from build123d import *

# Parameters (mm, degrees)
SKETCH2_W           = 124
SKETCH2_H           = 62
SKETCH2_R           = 1.55
SKETCH2_W_2         = 26.6
SKETCH2_H_2         = 14.6
SKETCH2_R_2         = 3.75
SKETCH2_R_3         = 8.3
SKETCH2_R_4         = 8.2
BOSS_EXTRUDE1_DEPTH = 4
CHAMFER1_SIZE       = 1.5
CHAMFER2_SIZE       = 1
SKETCH2_3_R         = 0.8
BOSS_EXTRUDE2_DEPTH = 3.5
FILLET1_R           = 0.8
CUT_EXTRUDE1_START  = 3
SKETCH2_4_W         = 28
SKETCH2_4_H         = 28.35
SKETCH2_4_R         = 0.8
SKETCH2_4_W_2       = 26.6
SKETCH2_4_H_2       = 14.6
CUT_EXTRUDE1_DEPTH  = 3
CHAMFER3_SIZE       = 1
SKETCH2_5_W         = 13.2
SKETCH2_5_H         = 14
CUT_EXTRUDE4_DEPTH  = 1.5


with BuildPart() as part:
    # Sketch2 → Boss-Extrude1 (new body)
    with BuildSketch(Plane(origin=(0, 0, 0), x_dir=(1, 0, 0), z_dir=(0, 1, 0))):
        with Locations((62, 31)):
            Rectangle(SKETCH2_W, SKETCH2_H)
        with Locations(Location((4.5, 4.5, 0), (0, 0, 270))):
            Circle(SKETCH2_R, mode=Mode.SUBTRACT)
        with Locations(Location((119.5, 4.5, 0), (0, 0, 270))):
            Circle(SKETCH2_R, mode=Mode.SUBTRACT)
        with Locations((28.239743387, 41.89740921)):
            Rectangle(SKETCH2_W_2, SKETCH2_H_2, mode=Mode.SUBTRACT)
        with Locations(Location((4.5, 57.5, 0), (0, 0, 270))):
            Circle(SKETCH2_R, mode=Mode.SUBTRACT)
        with Locations(Location((67.078277823, 40.203161161, 0), (0, 0, 270))):
            Circle(SKETCH2_R_2, mode=Mode.SUBTRACT)
        with Locations(Location((119.5, 57.5, 0), (0, 0, 270))):
            Circle(SKETCH2_R, mode=Mode.SUBTRACT)
        with Locations(Location((102.593331931, 31, 0), (0, 0, 270))):
            Circle(SKETCH2_R_3, mode=Mode.SUBTRACT)
        with BuildLine():
            ThreePointArc((79.454234541, 11.660627935), (68.529234541, 14.839562505), (79.454234541, 18.018497075))
            Line((79.454234541, 18.018497075), (79.454234541, 11.660627935))
        make_face(mode=Mode.SUBTRACT)
        with Locations(Location((48.846547615, 14.839562505, 0), (0, 0, 270))):
            Circle(SKETCH2_R_4, mode=Mode.SUBTRACT)
        with Locations(Location((23.171087178, 14.839562505, 0), (0, 0, 270))):
            Circle(SKETCH2_R_4, mode=Mode.SUBTRACT)
    extrude(amount=BOSS_EXTRUDE1_DEPTH)

    # Chamfer1
    chamfer1_edges = [part.edges().sort_by_distance(p)[0] for p in [
        (62, 4, 0),
        (124, 4, -31),
        (62, 4, -62),
        (0, 4, -31),
    ]]
    chamfer(chamfer1_edges, length=CHAMFER1_SIZE)

    # Chamfer2
    chamfer2_edges = [part.edges().sort_by_distance(p)[0] for p in [
        (119.5, 0, -59.05),
        (4.5, 4, -6.05),
        (119.5, 4, -59.05),
        (119.5, 4, -6.05),
        (4.5, 4, -59.05),
    ]]
    chamfer(chamfer2_edges, length=CHAMFER2_SIZE)

    # Sketch2<3> → Boss-Extrude2 (add)
    with BuildSketch(Plane(origin=(0, 0, 0), x_dir=(1, 0, 0), z_dir=(0, 1, 0))):
        with Locations(Location((16.679743387, 28.409287577, 0), (0, 0, 270))):
            Circle(SKETCH2_3_R)
        with Locations(Location((16.679743387, 51.709287577, 0), (0, 0, 270))):
            Circle(SKETCH2_3_R)
        with Locations(Location((39.799743387, 28.409287577, 0), (0, 0, 270))):
            Circle(SKETCH2_3_R)
        with Locations(Location((39.799743387, 51.709287577, 0), (0, 0, 270))):
            Circle(SKETCH2_3_R)
    extrude(amount=-BOSS_EXTRUDE2_DEPTH)

    # Fillet1
    fillet1_edges = [part.edges().sort_by_distance(p)[0] for p in [
        (39.799743387, -3.5, -29.209287577),
        (39.799743387, -3.5, -52.509287577),
        (16.679743387, -3.5, -29.209287577),
        (16.679743387, -3.5, -52.509287577),
    ]]
    fillet(fillet1_edges, radius=FILLET1_R)

    # Sketch2<4> → Cut-Extrude1 (cut)
    with BuildSketch(Plane(origin=(0, 0, 0), x_dir=(1, 0, 0), z_dir=(0, 1, 0)).offset(CUT_EXTRUDE1_START)):
        with Locations((28.239743387, 39.62240921)):
            Rectangle(SKETCH2_4_W, SKETCH2_4_H)
        with Locations(Location((16.679743387, 51.709287577, 0), (0, 0, 270))):
            Circle(SKETCH2_4_R, mode=Mode.SUBTRACT)
        with Locations(Location((16.679743387, 28.409287577, 0), (0, 0, 270))):
            Circle(SKETCH2_4_R, mode=Mode.SUBTRACT)
        with Locations(Location((39.799743387, 28.409287577, 0), (0, 0, 270))):
            Circle(SKETCH2_4_R, mode=Mode.SUBTRACT)
        with Locations(Location((39.799743387, 51.709287577, 0), (0, 0, 270))):
            Circle(SKETCH2_4_R, mode=Mode.SUBTRACT)
        with Locations((28.239743387, 41.89740921)):
            Rectangle(SKETCH2_4_W_2, SKETCH2_4_H_2, mode=Mode.SUBTRACT)
    extrude(amount=-CUT_EXTRUDE1_DEPTH, mode=Mode.SUBTRACT)

    # Chamfer3
    chamfer3_edges = [part.edges().sort_by_distance(p)[0] for p in [
        (28.239743387, 4, -34.59740921),
        (41.539743387, 4, -41.89740921),
        (14.939743387, 4, -41.89740921),
        (28.239743387, 4, -49.19740921),
    ]]
    chamfer(chamfer3_edges, length=CHAMFER3_SIZE - 0.0001)  # a hair under: the kernel refuses the full size

    # Sketch2<5> → Cut-Extrude4 (cut)
    with BuildSketch(Plane(origin=(0, 0, 0), x_dir=(1, 0, 0), z_dir=(0, 1, 0))):
        with Locations((67.078277823, 40.203161161)):
            Rectangle(SKETCH2_5_W, SKETCH2_5_H)
    extrude(amount=CUT_EXTRUDE4_DEPTH, mode=Mode.SUBTRACT)


solid = part.part
The listing builds one solid part. Answer for the finished solid, in the listing's coordinates (mm). A direction names the side the tool comes from. Give positions to 0.01 mm unless a question says otherwise; leave off trailing zeros. Write each loop counter-clockwise with the first axis right and the second up, starting at its lowest first coordinate (ties: lowest second). Pieces come first, ordered by that corner, then holes. Notation, with made-up numbers: (19, 53.5) - (63, 53.5) arc R21 cw to (63, 83.5) - close; hole circle Ø9 at (-29.75, 31). An arc over 180 degrees is marked (long way). One line per question, with ' | ' between items. Start each with the question number.
1. Section D-D, the plane z = -13.5 is taken. Determine the outline of the cut face in (x, y), then the cut area to 3 significant figures.
2. Section B-B, the plane z = -4.5 is taken. Determine the outline of the cut face in (x, y), then the cut area to 3 significant figures.
3. Straight lines are drawn through the part: line 1 (X direction, y = 1.65, z = -4.5); line 2 (Z direction, x = 74.5, y = 1.75); line 3 (Z direction, x = 30.5, y = 2.5). For each, find the intervals that lie inside material, in ascending order.
4. For faces 5 (the face through (118.125, 1.986, -56.785)), 6 (the face through (42.24, 2, -39)), determine the directions among +Z, -Z, +X, -X, +Y, -Y from which every point of the face is accessible in a straight line to the end or side of a thin tool.
5. Determine the mould class of faces 1 (the face through (124, 1, -31)), 2 (the face through (0, 1, -31)), 3 (the face through (61, 4, -31)), 4 (the face through (4.966, 1.479, -56.022)) for opening direction X: +X half, -X half, draft (parallel to the pull), parting line (faces both ways), or undercut.
6. Section C-C, the plane z = -30.5 is taken. Determine the outline of the cut face in (x, y), then the cut area to 3 significant figures.
7. Given P1, Ø12, axis at x = 40, z = -42.5, coming from the -Y side; P2, Ø2.5, axis at x = 4.5, z = -57.5, coming from the +Y side; P3, Ø4, axis at x = 119.5, z = -4.5, coming from the +Y side, each flat-ended and moving along its own axis, determine where each tip first touches the part or whether it passes through.
Result:
1) outline: (0, 0) - (15.08, 0) - (15.08, 4) - (1.5, 4) - (0, 2.5) - close; (31.26, 0) - (40.76, 0) - (40.76, 4) - (31.26, 4) - close; (56.94, 0) - (68.68, 0) - (68.68, 4) - (56.94, 4) - close; (79.45, 0) - (124, 0) - (124, 2.5) - (122.5, 4) - (79.45, 4) - close | area: 321 mm2
2) outline: (0, 0) - (2.95, 0) - (2.95, 3) - (1.95, 4) - (1.5, 4) - (0, 2.5) - close; (6.05, 0) - (117.95, 0) - (117.95, 3) - (116.95, 4) - (7.05, 4) - (6.05, 3) - close; (121.05, 0) - (124, 0) - (124, 2.5) - (122.5, 4) - (122.05, 4) - (121.05, 3) - close | area: 467 mm2
3) line 1: x = 0 to 2.95, 6.05 to 117.95, 121.05 to 124 | line 2: z = -62 to -20.76, -8.91 to 0 | line 3: z = -62 to -53.8, -25.45 to -18.52, -11.16 to 0
4) face 5: +Y, -Y | face 6: -Y
5) face 1: +X half | face 2: -X half | face 3: draft | face 4: undercut
6) outline: (0, 0) - (14.24, 0) - (14.24, 3) - (42.24, 3) - (42.24, 0) - (94.31, 0) - (94.31, 4) - (1.5, 4) - (0, 2.5) - close; (110.88, 0) - (124, 0) - (124, 2.5) - (122.5, 4) - (110.88, 4) - close | area: 343 mm2
7) P1: stops at y = 0 | P2: passes through | P3: stops at y = 3.45
